Source: CAD feature listing. Evaluate the final solid. Frame: model axes, mm. A direction names the side the tool comes from. Coordinates: 2 decimals unless noted, no trailing zeros. Write each loop counter-clockwise with the first axis right and the second up, starting at its lowest first coordinate (ties: lowest second). Pieces come first, ordered by that corner, then holes. Notation, with made-up numbers: (22.5, -4) - (55.5, -4) arc R17 ccw to (55.5, 4) - close; hole circle Ø1 at (69.5, 53.25). An arc over 180 degrees is marked (long way). One line per item, written item: value.
from build123d import *

# Parameters (mm, degrees)
EXTRUDE_THIN1_DEPTH  = 38.1
FILLET4_R            = 2.54
CUT_EXTRUDE1_REACH   = 49.805
SKETCH2_R            = 2.54
LPATTERN1_COUNT      = 5
LPATTERN1_PITCH      = 9.525
LPATTERN1_COUNT_DIR2 = 4
LPATTERN1_PITCH_DIR2 = 9.906


# Read off the part's stored shape, not the designer's step: Extrude-Thin1
with BuildPart() as part:
    # Extrude-Thin1 outline → Extrude-Thin1 (new body)
    with BuildSketch(Plane(origin=(0, 0, 0), x_dir=(1, 0, 0), z_dir=(0, 1, 0))):
        with BuildLine():
            Line((-22.861781044, -2.54), (23.293769416, -2.54))
            add(Edge.make_bspline(
                [(23.293769416, -2.54), (23.690788447, -2.589711931), (24.035397246, -2.670596213), (24.637666039, -2.878281595), (24.89574137, -3.004419147), (25.360322074, -3.302989633), (25.56786948, -3.475729285), (25.960337052, -3.895478718), (26.145315815, -4.143465548), (26.319262748, -4.44481044)],
                knots=[0, 0, 0, 0, 0.25, 0.25, 0.5, 0.5, 0.75, 0.75, 1, 1, 1, 1], degree=3))
            Line((26.319262748, -4.44481044), (28.519076705, -3.175))
            add(Edge.make_bspline(
                [(23.439076705, 0), (26.898166275, -0.366941984), (28.519076705, -3.175)],
                knots=[0, 0, 0, 1, 1, 1], degree=2))
            Line((23.439076705, 0), (-23.042923295, 0))
            add(Edge.make_bspline(
                [(-28.122923295, -3.175), (-26.434307868, -0.449952866), (-23.042923295, 0)],
                knots=[0, 0, 0, 1, 1, 1], degree=2))
            Line((-28.122923295, -3.175), (-25.963846277, -4.512903744))
            add(Edge.make_bspline(
                [(-25.963846277, -4.512903744), (-25.780355431, -4.216790612), (-25.585675804, -3.967832958), (-25.171704683, -3.539458263), (-24.952325189, -3.359368522), (-24.467192442, -3.046070455), (-24.200731304, -2.912638022), (-23.592393193, -2.689707924), (-23.250169649, -2.600640103), (-22.861781044, -2.54)],
                knots=[0, 0, 0, 0, 0.25, 0.25, 0.5, 0.5, 0.75, 0.75, 1, 1, 1, 1], degree=3))
        make_face()
    extrude(amount=EXTRUDE_THIN1_DEPTH)

    # Fillet4
    fillet4_edges = [part.edges().sort_by_distance(p)[0] for p in [
        (27.419169727, 38.1, 3.80990522),
        (27.419169727, 0, 3.80990522),
        (-27.043384786, 0, 3.843951872),
        (-27.043384786, 38.1, 3.843951872),
    ]]
    fillet(fillet4_edges, radius=FILLET4_R)

    # Sketch2 → Cut-Extrude1 (cut, up to next)
    with BuildSketch(Plane(origin=(0, 0, 0), x_dir=(-1, 0, 0), z_dir=(0, 0, -1)), mode=Mode.PRIVATE) as cut_extrude1_sk1:
        with Locations((18.890510813, 33.960005412)):
            Circle(SKETCH2_R)
    cut_extrude1_tool1 = extrude(cut_extrude1_sk1.sketch, amount=-CUT_EXTRUDE1_REACH, mode=Mode.PRIVATE) & part.part
    cut_extrude1 = cut_extrude1_tool1.solids().sort_by_distance((-18.890511, 33.960005, 0))[0]
    add(cut_extrude1, mode=Mode.SUBTRACT)

    # LPattern1: Cut-Extrude1 5 × 4
    with Locations(*[(i * LPATTERN1_PITCH, -j * LPATTERN1_PITCH_DIR2, 0) for i in range(LPATTERN1_COUNT) for j in range(LPATTERN1_COUNT_DIR2) if (i, j) != (0, 0)]):
        add(cut_extrude1, mode=Mode.SUBTRACT)


solid = part.part
1) Section query B-B on y = 23. State how many separate pieces and enclosed holes the cut face has, then the cut area to 3 significant figures.
Values found:
separate pieces: 6
enclosed holes: 0
area: 84.3 mm2
2) Draft query along X for faces 3 (the flat face through (1, 19, 0)), 4 (the cylindrical face through (-26.6, 37.336, 3.267)), 5 (the cylindrical face through (0.71, 11.67, 1.25)). Return one class per face: released by +X, released by -X, zero draft, split by the parting line, or undercut.
Values found:
face 3: zero draft
face 4: released by -X
face 5: undercut
3) Reachability of faces 1 (the cylindrical face through (2.18, 2.7, 1.25)), 2 (the flat face through (0, 19, 2.54)) from +Z, -Z, +X, -X, +Y, -Y: full face, straight path, thin tool, end or side. Return the list, or none.
Values found:
face 1: +Z, -Z
face 2: +Z, +Y, -Y
4) Section query A-A on x = 0.5. Output: boundary loops of the cut face in (y, z).
Values found:
outline: (0, 0) - (1.72, 0) - (1.72, 2.54) - (0, 2.54) - close; (6.76, 0) - (11.63, 0) - (11.63, 2.54) - (6.76, 2.54) - close; (16.67, 0) - (21.54, 0) - (21.54, 2.54) - (16.67, 2.54) - close; (26.57, 0) - (31.44, 0) - (31.44, 2.54) - (26.57, 2.54) - close; (36.48, 0) - (38.1, 0) - (38.1, 2.54) - (36.48, 2.54) - close
5) Section query C-C on x = 13.5. Output: boundary loops of the cut face in (y, z).
Values found:
outline: (0, 0) - (38.1, 0) - (38.1, 2.54) - (0, 2.54) - close
6) Contact query for flat-ended pins moving along their axis: P1, Ø11.5, axis at x = 3, y = 12, coming from the +Z side; P2, Ø1.5, axis at y = 12, z = 0.5, coming from the -X side. Output: stop coordinate, or through.
Values found:
P1: z = 2.54
P2: x = -26.35
7) Material intervals for line 1 (Y direction, x = 2, z = 1.05); line 2 (Y direction, x = 17, z = 1.8); line 3 (X direction, y = 24.5, z = 1.1), sorted ascending.
Values found:
line 1: 0 to 2.49, 5.99 to 12.4, 15.9 to 22.3, 25.8 to 32.21, 35.71 to 38.1
line 2: 0 to 2.99, 5.49 to 12.9, 15.4 to 22.8, 25.31 to 32.71, 35.21 to 38.1
line 3: -26.14 to -21.39, -16.39 to -11.87, -6.86 to -2.34, 2.66 to 7.18, 12.19 to 16.71, 21.71 to 26.63
